Study the drawing (mm; zero at the part's minimum x, y, z) and answer. A direction names the side the tool comes from. Coordinates: 2 decimals unless noted, no trailing zeros. Write each loop counter-clockwise with the first axis right and the second up, starting at its lowest first coordinate (ties: lowest second). Pieces come first, ordered by that corner, then holes. Notation, with made-up numbers: (61.25, -11) - (120.25, -11) arc R26 ccw to (120.25, 6) - close; hole circle Ø11 at (76, 47). An arc over 180 degrees is marked (long way). One line per item, written item: value.
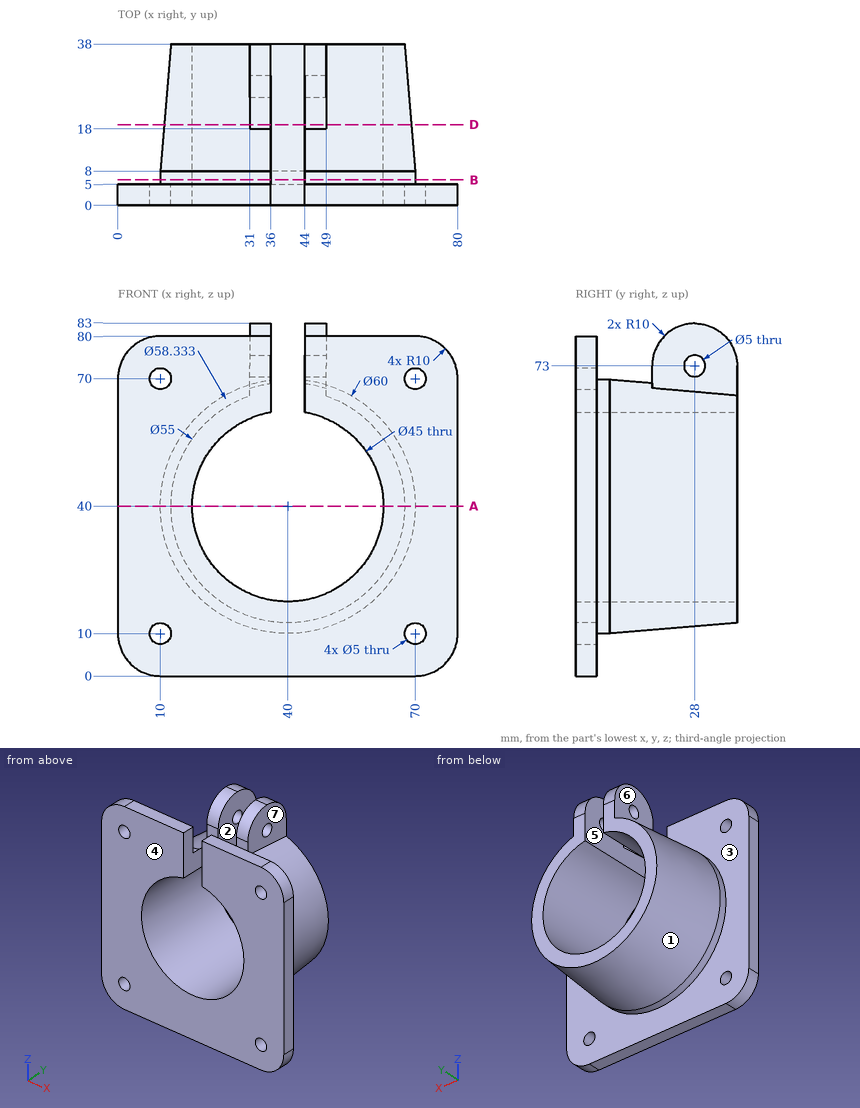
Item 1: Section D-D, the plane y = 19 is taken. Determine the outline of the cut face in (x, z), then the cut area to 3 significant figures.
Evaluation:
outline: (31, 67.66) arc R29.08 ccw (long way) to (49, 67.66) - (49, 77.36) - (44, 77.36) - (44, 62.14) arc R22.5 cw (long way) to (36, 62.14) - (36, 77.36) - (31, 77.36) - close
area: 1,100 mm2
Item 2: Determine the mould class of the marked faces 1, 2 and 3 for opening direction X: +X half, -X half, draft (parallel to the pull), parting line (faces both ways), or undercut.
Evaluation:
face 1: parting line
face 2: undercut
face 3: draft
Item 3: Section A-A, the plane z = 40 is taken. Determine the outline of the cut face in (x, y), then the cut area to 3 significant figures.
Evaluation:
outline: (0, 0) - (17.5, 0) - (17.5, 38) - (12.5, 38) - (10, 8) - (10, 5) - (0, 5) - close; (62.5, 0) - (80, 0) - (80, 5) - (70, 5) - (70, 8) - (67.5, 38) - (62.5, 38) - close
area: 595 mm2
Item 4: Consider probe 1 along X at (y, z) = (2.9, 10); probe 2 along X at (y, z) = (3.5, 64); probe 3 along X at (y, z) = (2.5, 69). Determine where each line is inside the solid, lowest interval first.
Evaluation:
probe 1: x = 0 to 7.5, 12.5 to 67.5, 72.5 to 80
probe 2: x = 0 to 36, 44 to 80
probe 3: x = 0 to 7.71, 12.29 to 36, 44 to 67.71, 72.29 to 80
Item 5: Section B-B, the plane y = 6 is taken. Determine the outline of the cut face in (x, z), then the cut area to 3 significant figures.
Evaluation:
outline: (36, 62.14) - (36, 69.73) arc R30 ccw (long way) to (44, 69.73) - (44, 62.14) arc R22.5 cw (long way) to start
area: 1,180 mm2
Item 6: Which of the six approach directions +Z, -Z, +X, -X, +Y, -Y give full straight-line access (tool end or side, diameter ignored) to the marked faces 4, 5, 6 and 7?
Evaluation:
face 4: +Z, -Z, +X, -X, -Y
face 5: +Z, +Y, -Y
face 6: +Z, -X, +Y
face 7: +Z, +X, +Y
Item 7: Given pin 1 (1.5 mm diameter, centred on y = 18, z = 70.5, fed in from +X); pin 2 (6.5 mm diameter, centred on y = 28, z = 73, fed in from -X); pin 3 (8 mm diameter, centred on x = 23, y = 23.5, fed in from +Z), each flat-ended and moving along its own axis, determine where each tip first touches the part or whether it passes through.
Evaluation:
pin 1: stops at x = 49
pin 2: stops at x = 31
pin 3: stops at z = 65.63
